from build123d import *

# Parameters (mm, degrees)
ESBO_O1_R                = 55
RESSALTO_EXTRUS_O1_DEPTH = 8
RESSALTO_EXTRUS_O2_DEPTH = 4
ESBO_O3_R                = 1.65
CORTE_EXTRUS_O1_DEPTH    = 3
ESBO_O4_R                = 2.9
CORTE_EXTRUS_O2_DEPTH    = 5
FILETE1_R                = 4


with BuildPart() as part:
    # Esboço1 → Ressalto-extrusão1 (new body)
    with BuildSketch(Plane.XY):
        Circle(ESBO_O1_R)
    extrude(amount=RESSALTO_EXTRUS_O1_DEPTH)

    # Esboço2 → Ressalto-extrusão2 (add)
    with BuildSketch(Plane.XY.offset(8)):
        with BuildLine():
            Line((-44.830681458, 3.9), (-54.861553022, 3.9))
            ThreePointArc((-54.861553022, 3.9), (-55, 0), (-54.861553022, -3.9))
            Line((-54.861553022, -3.9), (-44.830681458, -3.9))
            ThreePointArc((-44.830681458, -3.9), (45, 0), (-44.830681458, 3.9))
        make_face()
    extrude(amount=RESSALTO_EXTRUS_O2_DEPTH)

    # Esboço3 → Corte-extrusão1 (cut)
    with BuildSketch(Plane.XY.offset(8)):
        with Locations((2.2845e-05, -50)):
            Circle(ESBO_O3_R)
        with Locations((-43.301247344, 25)):
            Circle(ESBO_O3_R)
        with Locations((43.301293034, 25)):
            Circle(ESBO_O3_R)
    extrude(amount=-CORTE_EXTRUS_O1_DEPTH, mode=Mode.SUBTRACT)

    # Esboço4 → Corte-extrusão2 (cut)
    with BuildSketch(Plane.XY.offset(5)):
        with Locations((-43.301247344, 25)):
            Circle(ESBO_O4_R)
        with Locations((43.301293034, 25)):
            Circle(ESBO_O4_R)
        with Locations((2.2845e-05, -50)):
            Circle(ESBO_O4_R)
    extrude(amount=-CORTE_EXTRUS_O2_DEPTH, mode=Mode.SUBTRACT)

    # Filete1
    # the kernel refuses this fillet: 4 mm, written as the material it takes off along each edge
    with BuildSketch(Plane(origin=(0, 0, 0), x_dir=(1, 0, 0), z_dir=(0, -1, 0))) as filete1_piece_1:
        with BuildLine():
            CenterArc((55 - FILETE1_R, FILETE1_R), FILETE1_R, 270, 90)
            Line((55 - FILETE1_R, 0), (55, 0))
            Line((55, 0), (55, FILETE1_R))
        make_face()
    revolve(axis=Axis((0, 0, 0), (0, 0, 1)), mode=Mode.SUBTRACT)


solid = part.part
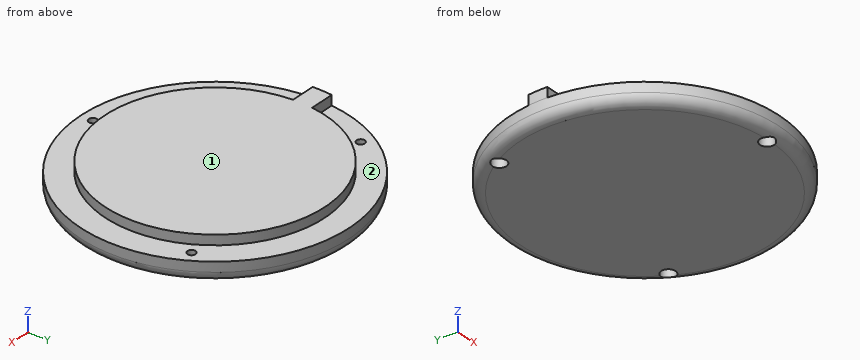
Check sheet for the modelled part. Datum: model origin and axes. Units: mm. Face numbers are marked on the shaded views. A direction names the side the tool comes from. Give positions to 0.01 mm unless a question says otherwise; leave off trailing zeros. Write each loop counter-clockwise with the first axis right and the second up, starting at its lowest first coordinate (ties: lowest second). Pieces come first, ordered by that corner, then holes. Notation, with made-up numbers: (22, 35) -> (39, 35) arc R20 ccw to (39, 59) -> close; hole circle Ø1 at (-16.5, 25). An arc over 180 degrees is marked (long way). Use one line per item in the form item = value. Start each with the question number.
1. Thickness scan on line 1 along X through (y, z) = (25, 3); line 2 along X through (y, z) = (25, 1.45); line 3 along Z through (x, y) = (0, 49.5). Record the ranges inside material, lowest first. Write a range as from..to.
2. Access from +Z, -Z, +X, -X, +Y, -Y to the whole of each face (thin tool, end or side, straight path). Record for the marked faces 1 and 2.
3. Go/stop test with flat-tipped pins: P1, Ø1.7, axis at x = -1, y = -49.5, coming from the -Z side; P2, Ø6.5, axis at x = -43.3, y = 25, coming from the +Z side; P3, Ø2, axis at x = -51, z = 10.5, coming from the +Y side. Record where each tip stops, or that it passes through.
4. Section check B-B (x = 0). Record the cut outline in (y, z), and give its area (3 significant figures).
5. Section check D-D (z = 2). Record the cut outline in (x, y), and give its area (3 significant figures).
6. Section check A-A (y = 0). Record the cut outline in (x, z), and give its area (3 significant figures).
7. Section check C-C (z = 10). Record the cut outline in (x, y), and give its area (3 significant figures).
Conclusion:
q1.line_1 = -48.85..-46.2, -40.4..40.4, 46.2..48.85
q1.line_2 = -47.96..-46.2, -40.4..40.4, 46.2..47.96
q1.line_3 = 0..8
q2.face_1 = +Z, +X, -X, +Y, -Y
q2.face_2 = +Z
q3.P1 = 5
q3.P2 = 8
q3.P3 = 3.9
q4.outline = (-55, 4) arc R4 ccw to (-52.9, 0.48) -> (-52.9, 5) -> (-51.65, 5) -> (-51.65, 8) -> (-55, 8) -> close; (-48.35, 5) -> (-47.1, 5) -> (-47.1, 0) -> (51, 0) arc R4 ccw to (55, 4) -> (55, 8) -> (45, 8) -> (45, 12) -> (-45, 12) -> (-45, 8) -> (-48.35, 8) -> close
q4.area = 1,190 mm²
q5.outline = circle Ø108.93 at (0, 0); hole circle Ø5.8 at (-43.3, 25); hole circle Ø5.8 at (0, -50); hole circle Ø5.8 at (43.3, 25)
q5.area = 9,240 mm²
q6.outline = (-55, 4) arc R4 ccw to (-51, 0) -> (51, 0) arc R4 ccw to (55, 4) -> (55, 8) -> (45, 8) -> (45, 12) -> (-55, 12) -> close
q6.area = 1,270 mm²
q7.outline = (-54.86, -3.9) -> (-44.83, -3.9) arc R45 ccw (long way) to (-44.83, 3.9) -> (-54.86, 3.9) arc R55 ccw to start
q7.area = 6,440 mm²
